Geometry: see drawing. Coordinates: mm, zero at the bounding-box minimum. Coordinates: 2 decimals unless noted, no trailing zeros. Order: outer loops, then holes, each group sorted by start corner. A loop starts at its lowest first (then second) coordinate and runs counter-clockwise, first axis right, second up. Notation, with made-up numbers: M 59.25,68.5 L 87.25,68.5 A28 cw 87.25,102.5 Z; hole C 54,6.5 d8. An arc over 180 degrees is marked long. One line per item, written item: value.
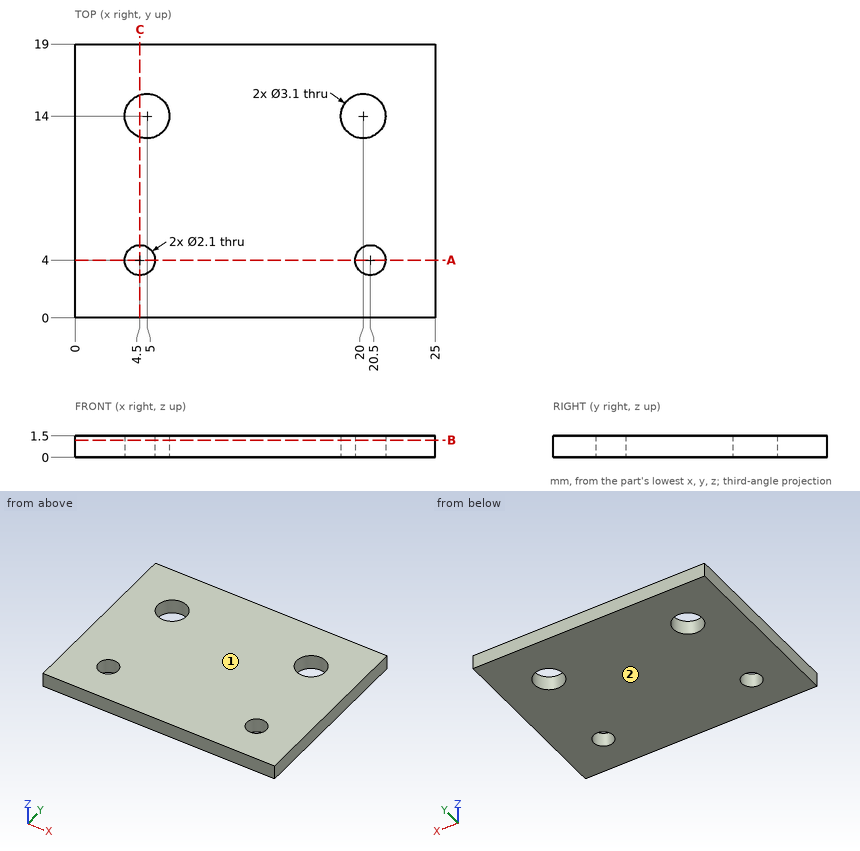
(1) Ray query, line 1 (X direction, y = 14, z = 0.85); line 2 (X direction, y = 4, z = 0.4); line 3 (Y direction, x = 4.5, z = 0.65). Return the intervals inside material, ascending. Write a range as from..to.
Data:
line 1: x = 0..3.45, 6.55..18.45, 21.55..25
line 2: x = 0..3.45, 5.55..19.45, 21.55..25
line 3: y = 0..2.95, 5.05..12.53, 15.47..19
(2) Cut plane C-C on x = 4.5. Output: boundary loops of the cut face in (y, z).
Data:
outline: M 0,0 L 2.95,0 L 2.95,1.5 L 0,1.5 Z; M 5.05,0 L 12.53,0 L 12.53,1.5 L 5.05,1.5 Z; M 15.47,0 L 19,0 L 19,1.5 L 15.47,1.5 Z
(3) Cut plane B-B on z = 1.2. Output: boundary loops of the cut face in (x, y).
Data:
outline: M 0,0 L 25,0 L 25,19 L 0,19 Z; hole C 4.5,4 d2.1; hole C 5,14 d3.1; hole C 20,14 d3.1; hole C 20.5,4 d2.1
(4) Cut plane A-A on y = 4. Output: boundary loops of the cut face in (x, z).
Data:
outline: M 0,0 L 3.45,0 L 3.45,1.5 L 0,1.5 Z; M 5.55,0 L 19.45,0 L 19.45,1.5 L 5.55,1.5 Z; M 21.55,0 L 25,0 L 25,1.5 L 21.55,1.5 Z
(5) Draft query along Z for the marked faces 1 and 2. Return one class per face: released by +Z, released by -Z, zero draft, split by the parting line, or undercut.
Data:
face 1: released by +Z
face 2: released by -Z
